Drawing for the job (mm, zero at the part's lowest x, y, z). A direction names the side the tool comes from. Give positions to 0.01 mm unless a question says otherwise; leave off trailing zeros. Order: outer loops, then holes, each group sorted by start corner. A loop starts at its lowest first (then second) coordinate and runs counter-clockwise, first axis right, second up. Notation, with made-up numbers: (-28, -7) -> (-8, -7) arc R10 ccw to (-8, -2) -> close; hole circle Ø10 at (70.25, 30). An arc over 180 degrees is marked (long way). One line per item, written item: value. Start each with the question number.
(1) Saw through at B-B on z = 9. Give the cut face in (x, y), plus the area to 3 significant figures.
(2) Pin check, flat tips, straight feed: pin 1 (1.6 mm diameter, centred on x = 14.2, z = 12, fed in from -Y); pin 2 (3 mm diameter, centred on x = 7.5, z = 13, fed in from -Y); pin 3 (6 mm diameter, centred on x = 12.5, z = 14.5, fed in from +Y); pin 4 (4 mm diameter, centred on y = 7, z = 4.5, fed in from +X). Stop position of each tip, or through.
(3) Probe line 1 (Z direction, x = 9, y = 1.8) (3 decimals); line 2 (X direction, y = 2.1, z = 12) (1 decimal); line 3 (Y direction, x = 9.25, z = 5). List the from-to ranges inside material, lowest first.
(4) Which spindle directions (+Z, -Z, +X, -X, +Y, -Y) get a long thin tool onto all of the face, cutting with end or side? Do the marked faces 1 and 2. Say none if no direction does.
(5) Two-plate mould, pull along X, no slides. Class the marked faces 3, 4 and 5: +X half, -X half, draft (parallel to the pull), parting line (faces both ways), or undercut.
(6) Saw through at D-D on y = 11.75. Give the cut face in (x, z), plus the area to 3 significant figures.
(7) Saw through at A-A on x = 14. Give the cut face in (y, z), plus the area to 3 significant figures.
(8) Saw through at C-C on y = 2. Give the cut face in (x, z) (3 decimals), plus the area to 3 significant figures.
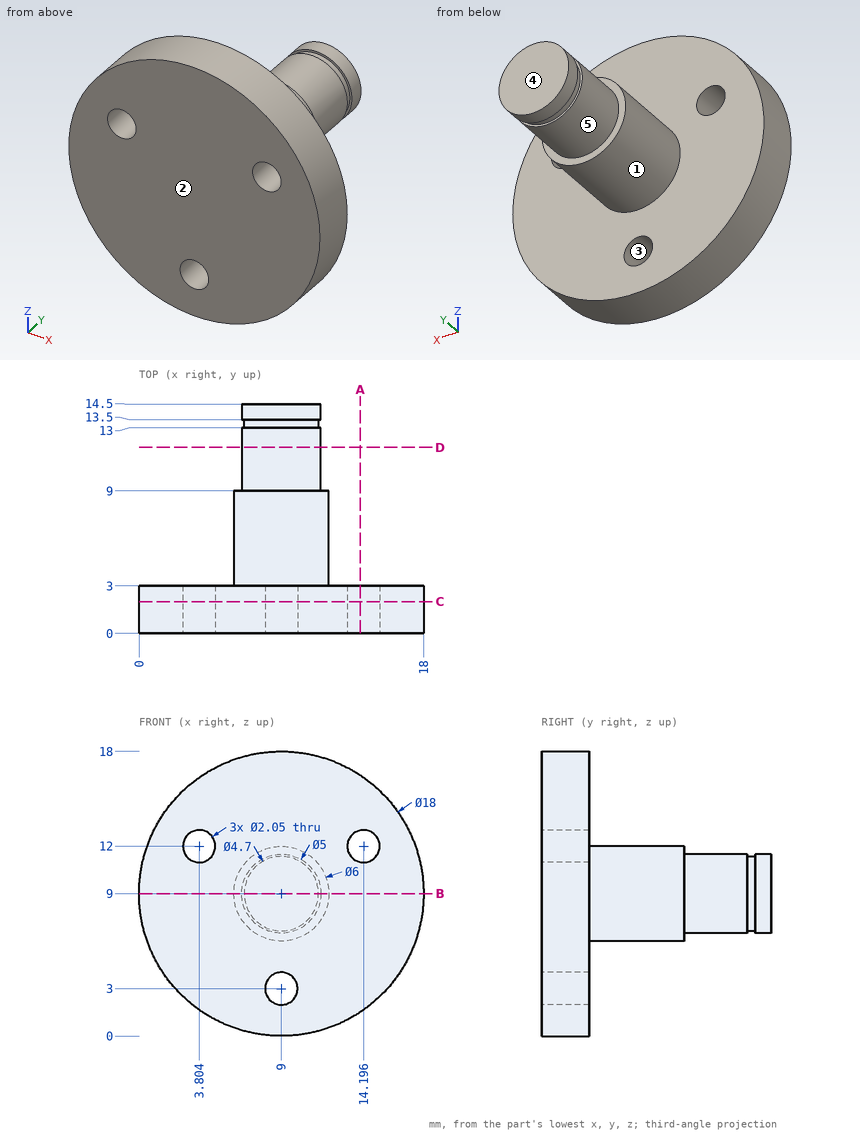
Results below:
1. outline: (0, 0) -> (18, 0) -> (18, 3) -> (12, 3) -> (12, 9) -> (11.5, 9) -> (11.5, 13) -> (11.35, 13) -> (11.35, 13.5) -> (11.5, 13.5) -> (11.5, 14.5) -> (6.5, 14.5) -> (6.5, 13.5) -> (6.65, 13.5) -> (6.65, 13) -> (6.5, 13) -> (6.5, 9) -> (6, 9) -> (6, 3) -> (0, 3) -> close
1. area: 117 mm²
2. pin 1: passes through
2. pin 2: stops at y = 0
2. pin 3: stops at y = 3
2. pin 4: stops at x = 10.66
3. line 1: z = 0 to 1.975, 4.025 to 18
3. line 2: x = 0.5 to 2.8, 4.8 to 13.2, 15.2 to 17.5
3. line 3: y = 0 to 3
4. face 1: +Y
4. face 2: +Z, -Z, +X, -X, -Y
5. face 3: undercut
5. face 4: draft
5. face 5: parting line
6. outline: circle Ø5 at (9, 9)
6. area: 19.6 mm²
7. outline: (0, 1.52) -> (3, 1.52) -> (3, 10.99) -> (0, 10.99) -> close; (0, 13.01) -> (3, 13.01) -> (3, 16.48) -> (0, 16.48) -> close
7. area: 38.9 mm²
8. outline: circle Ø18 at (9, 9); hole circle Ø2.05 at (3.804, 12); hole circle Ø2.05 at (9, 3); hole circle Ø2.05 at (14.196, 12)
8. area: 245 mm²
